Part print with two shaded views. Sizes in mm from the minimum x, y, z corner. A direction names the side the tool comes from. Round coordinates to 2 decimals unless told otherwise and drop trailing zeros. Loops run counter-clockwise (first coordinate to the right, second up) from the corner with the lowest first, then second, coordinate; pieces in that order, holes last.
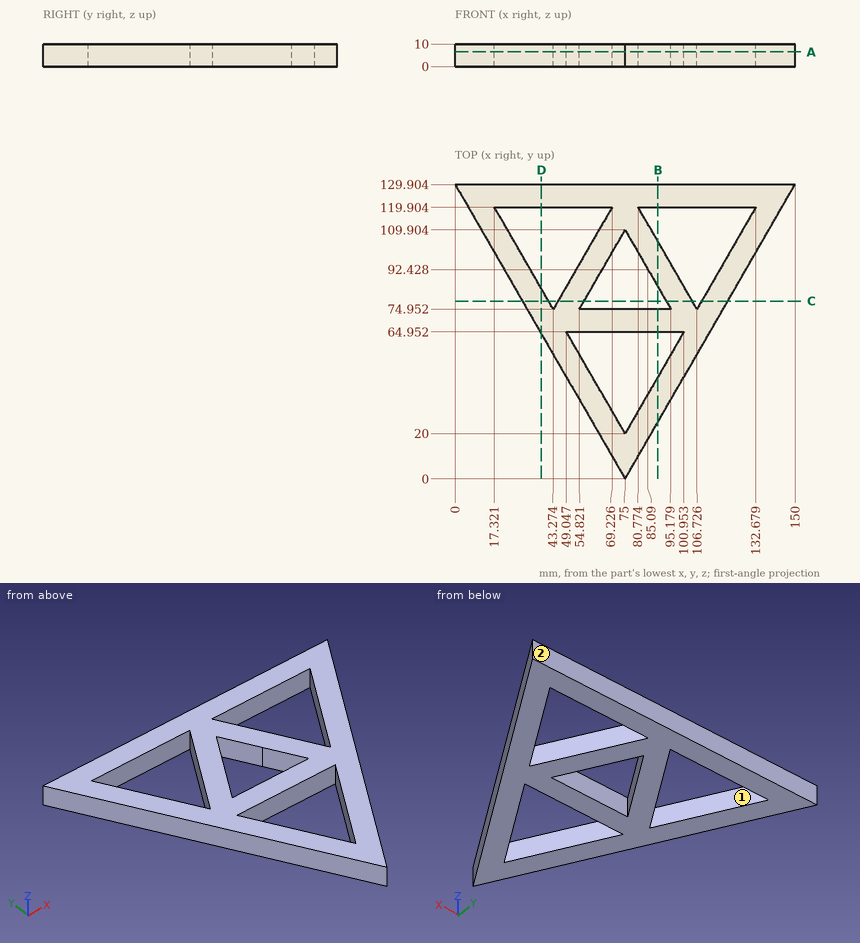
Item 1: 3-axis set-ups, long thin cutter, end or side, ignore diameter. For the marked faces 1 and 2: which of +Z, -Z, +X, -X, +Y, -Y reach the whole face in a straight line?
Verdict:
face 1: +Z, -Z
face 2: +Z, -Z, +X, -X, +Y
Item 2: Cut at D-D (x = 38). List the corners of the cut face in (y, z) (1 decimal), plus the area to 3 significant figures.
Verdict:
outline: (64.1, 0) - (84.1, 0) - (84.1, 10) - (64.1, 10) - close; (119.9, 0) - (129.9, 0) - (129.9, 10) - (119.9, 10) - close
area: 300 mm2
Item 3: Cut at C-C (y = 78.5). List the corners of the cut face in (x, z) (1 decimal).
Verdict:
outline: (29.7, 0) - (41.2, 0) - (41.2, 10) - (29.7, 10) - close; (45.3, 0) - (56.9, 0) - (56.9, 10) - (45.3, 10) - close; (93.1, 0) - (104.7, 0) - (104.7, 10) - (93.1, 10) - close; (108.8, 0) - (120.3, 0) - (120.3, 10) - (108.8, 10) - close
Item 4: Cut at B-B (x = 89.5). List the corners of the cut face in (y, z) (1 decimal), plus the area to 3 significant figures.
Verdict:
outline: (25.1, 0) - (45.1, 0) - (45.1, 10) - (25.1, 10) - close; (65, 0) - (75, 0) - (75, 10) - (65, 10) - close; (84.8, 0) - (104.8, 0) - (104.8, 10) - (84.8, 10) - close; (119.9, 0) - (129.9, 0) - (129.9, 10) - (119.9, 10) - close
area: 600 mm2
Item 5: Wall check: L1, parallel to X at y = 92, z = 9.5 (1 decimal); L2, parallel to X at y = 78, z = 2.75 (1 decimal); L3, parallel to X at y = 30.5, z = 9.25. Give the ranges that are in metal, low to high.
Verdict:
L1: x = 21.9 to 33.4, 53.1 to 64.7, 85.3 to 96.9, 116.6 to 128.1
L2: x = 30 to 41.5, 45 to 56.6, 93.4 to 105, 108.5 to 120
L3: x = 57.39 to 68.94, 81.06 to 92.61
Item 6: Flat gauge pins, fed straight in: P1, Ø1.5, axis at y = 114, z = 3, coming from the +X side; P2, Ø1.5, axis at y = 76, z = 4.5, coming from the +X side. Where does each tip first touch, or does it go through?
Verdict:
P1: stops at x = 141.25
P2: stops at x = 119.31
Item 7: Cut at A-A (z = 6.5). List the corners of the cut face in (x, y), plus the area to 3 significant figures.
Verdict:
outline: (0, 129.9) - (75, 0) - (150, 129.9) - close; hole (17.32, 119.9) - (43.27, 74.95) - (69.23, 119.9) - close; hole (49.05, 64.95) - (75, 20) - (100.95, 64.95) - close; hole (54.82, 74.95) - (95.18, 74.95) - (75, 109.9) - close; hole (80.77, 119.9) - (106.73, 74.95) - (132.68, 119.9) - close
area: 5,540 mm2
